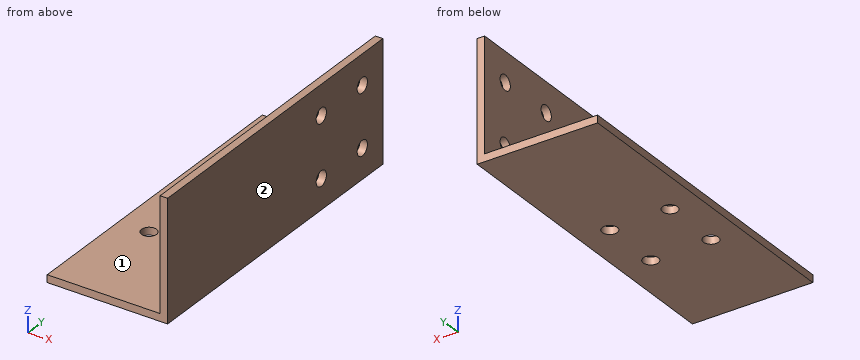
Autodesk Inventor part; units mm, degrees
ref_plane "YZ Plane" through (0, 0, 0) normal (1, 0, 0) x (0, 1, 0)
ref_plane "XZ Plane" through (0, 0, 0) normal (0, 1, 0) x (-1, 0, 0)
ref_plane "XY Plane" through (0, 0, 0) normal (0, 0, 1) x (1, 0, 0)
sketch "Sketch1" plane through (0, 0, 0) normal (0, 1, 0) x (-1, 0, 0)
  line L0 (0, 0) -> (3.175, 0)
  line L1 (3.175, 0) -> (3.175, 50.8)
  line L2 (3.175, 50.8) -> (0, 50.8)
  line L3 (0, 50.8) -> (0, 0)
  line L4 (0, 0) -> (50.8, 0)
  line L5 (50.8, 0) -> (50.8, 3.175)
  line L6 (50.8, 3.175) -> (0, 3.175)
  line L7 (0, 3.175) -> (0, 0)
  dimension "d0" = 3.175
  dimension "d1" = 50.8
  dimension "d2" = 50.8
  dimension "d3" = 3.175
extrude "Extrusion1" add sketch "Sketch1" along normal blind 133.35
sketch "Sketch2" plane through (0, 0, 50.8) normal (1, 0, 0) x (0, 0, -1)
  line L0 (0, 0) -> (50.8, 0)
  line L1 (50.8, 0) -> (50.8, 133.35)
  line L2 (0, 133.35) -> (50.8, 133.35)
  line L3 (0, 0) -> (0, 133.35)
  point P0 (12.7, 120.65)
  point P1 (38.1, 120.65)
  point P2 (38.1, 95.25)
  point P3 (12.7, 95.25)
  dimension "d6" = 12.7
  dimension "d7" = 12.7
  dimension "d8" = 12.7
  dimension "d9" = 12.7
  dimension "d10" = 12.7
  dimension "d11" = 12.7
  dimension "d12" = 38.1
  dimension "d13" = 38.1
hole "Hole1" at (0, 120.65, 38.1) at (0, 120.65, 12.7) at (0, 95.25, 12.7) at (0, 95.25, 38.1) direction (-1, 0, 0) diameter 6.35 end through all
sketch "Sketch3" plane through (0, 0, 0) normal (0, 0, -1) x (-1, 0, 0)
  line L0 (0, 133.35) -> (50.8, 133.35)
  line L1 (0, 0) -> (0, 133.35)
  line L2 (0, 0) -> (50.8, 0)
  line L3 (50.8, 0) -> (50.8, 133.35)
  point P0 (12.7, 69.85)
  point P1 (38.1, 69.85)
  point P2 (38.1, 44.45)
  point P3 (12.7, 44.45)
  dimension "d21" = 12.7
  dimension "d22" = 12.7
  dimension "d23" = 63.5
  dimension "d24" = 63.5
  dimension "d32" = 88.9
  dimension "d33" = 88.9
  dimension "d34" = 12.7
  dimension "d35" = 12.7
hole "Hole3" at (-12.7, 69.85, 0) at (-38.1, 69.85, 0) at (-38.1, 44.45, 0) at (-12.7, 44.45, 0) direction (0, 0, 1) diameter 6.35 end through all
properties part number "2x2 angle vertical right"
Input: part model. Units: mm. Frame: model coordinates. Face numbers are marked on the shaded views. A direction names the side the tool comes from. Give positions to 0.01 mm unless a question says otherwise; leave off trailing zeros. Order: outer loops, then holes, each group sorted by start corner. A loop starts at its lowest first (then second) coordinate and runs counter-clockwise, first axis right, second up. Notation, with made-up numbers: (-18.75, 12.5) - (33.25, 12.5) arc R31 ccw to (33.25, 50.5) - close; hole circle Ø10 at (-21, -32). An arc over 180 degrees is marked (long way). Use a Markdown table: item, result.
(1) Section query A-A (y = 69.85). Output: boundary loops of the cut face in (x, z) (3 decimals).
Computed values:
| item | result |
|---|---|
| outline | (-50.8, 0) - (-41.275, 0) - (-41.275, 3.175) - (-50.8, 3.175) - close; (-34.925, 0) - (-15.875, 0) - (-15.875, 3.175) - (-34.925, 3.175) - close; (-9.525, 0) - (0, 0) - (0, 50.8) - (-3.175, 50.8) - (-3.175, 3.175) - (-9.525, 3.175) - close |
(2) Section query C-C (z = 38.1). Output: boundary loops of the cut face in (x, y) (3 decimals), then the cut area to 3 significant figures.
Computed values:
| item | result |
|---|---|
| outline | (-3.175, 0) - (0, 0) - (0, 92.075) - (-3.175, 92.075) - close; (-3.175, 98.425) - (0, 98.425) - (0, 117.475) - (-3.175, 117.475) - close; (-3.175, 123.825) - (0, 123.825) - (0, 133.35) - (-3.175, 133.35) - close |
| area | 383 mm2 |
(3) Line query: line 1 (Z direction, x = -2.45, y = 120.65) (3 decimals); line 2 (Y direction, x = -38, z = 1); line 3 (X direction, y = 69.85, z = 1.75) (3 decimals). Output: solid intervals per line, ascending. Write a range as from..to.
Computed values:
| item | result |
|---|---|
| line 1 | z = 0..9.525, 15.875..34.925, 41.275..50.8 |
| line 2 | y = 0..41.28, 47.62..66.68, 73.02..133.35 |
| line 3 | x = -50.8..-41.275, -34.925..-15.875, -9.525..0 |
(4) Access query for the marked faces 1 and 2. Directions: +Z, -Z, +X, -X, +Y, -Y. A direction counts if a zero-diameter tool reaches every point of the face in a straight line with its end or side. Return the directions, or none.
Computed values:
| item | result |
|---|---|
| face 1 | +Z, -X, +Y, -Y |
| face 2 | +Z, -Z, +X, +Y, -Y |
(5) Pin query (flat end, axial travel): pin 1 (5 mm diameter, centred on x = -12.7, y = 69.85, fed in from +Z); pin 2 (2 mm diameter, centred on x = -11, y = 53.5, fed in from +Z) (3 decimals); pin 3 (10 mm diameter, centred on y = 95.25, z = 38.1, fed in from -X) (3 decimals). Return the tip coordinate at first contact, or that it passes through.
Computed values:
| item | result |
|---|---|
| pin 1 | passes through |
| pin 2 | stops at z = 3.175 |
| pin 3 | stops at x = -3.175 |
(6) Section query D-D (y = 112.5). Output: boundary loops of the cut face in (x, z) (3 decimals), then the cut area to 4 significant figures.
Computed values:
| item | result |
|---|---|
| outline | (-50.8, 0) - (0, 0) - (0, 50.8) - (-3.175, 50.8) - (-3.175, 3.175) - (-50.8, 3.175) - close |
| area | 312.5 mm2 |
(7) Section query B-B (x = -38.1). Output: boundary loops of the cut face in (y, z) (3 decimals), then the cut area to 3 significant figures.
Computed values:
| item | result |
|---|---|
| outline | (0, 0) - (41.275, 0) - (41.275, 3.175) - (0, 3.175) - close; (47.625, 0) - (66.675, 0) - (66.675, 3.175) - (47.625, 3.175) - close; (73.025, 0) - (133.35, 0) - (133.35, 3.175) - (73.025, 3.175) - close |
| area | 383 mm2 |
